from build123d import *

# Parameters (mm, degrees)
SKETCH_R          = 1.7
PAD_DEPTH         = 8
SKETCH001_R       = 1.5
POCKET_DEPTH      = 12.501
POCKET_DEPTH_BACK = -12.501
SKETCH002_R       = 3
POCKET001_DEPTH   = 2.25
SKETCH003_R       = 6
SKETCH003_R_2     = 3
POCKET002_DEPTH   = 4
SKETCH004_R       = 2.5
POCKET003_DEPTH   = 25.001
POCKET004_DEPTH   = 25.001
CHAMFER_SIZE      = 1
CHAMFER001_SIZE   = 1.5


with BuildPart() as part:
    # Sketch → Pad (new body)
    with BuildSketch(Plane.XY):
        Polygon((-12.5, 18), (-12.5, 0), (-12.5, -18), (0, -18), (12.5, -18), (12.5, 0), (12.5, 18), (0, 18), align=None)
        with Locations((6.5, -13)):
            Circle(SKETCH_R, mode=Mode.SUBTRACT)
        with Locations((-6.5, -13)):
            Circle(SKETCH_R, mode=Mode.SUBTRACT)
    extrude(amount=PAD_DEPTH)

    # Sketch001 → Pocket (cut, two sides)
    with BuildSketch(Plane.YZ) as pocket_sk:
        with Locations((0, 1.5)):
            Circle(SKETCH001_R)
    extrude(amount=-POCKET_DEPTH, mode=Mode.SUBTRACT)
    extrude(pocket_sk.sketch, amount=-POCKET_DEPTH_BACK, mode=Mode.SUBTRACT)

    # Sketch002 → Pocket001 (cut, symmetric)
    with BuildSketch(Plane.YZ):
        with Locations((0, 1.5)):
            Circle(SKETCH002_R)
    extrude(amount=POCKET001_DEPTH, both=True, mode=Mode.SUBTRACT)

    # Sketch003 → Pocket002 (cut, symmetric)
    with BuildSketch(Plane.YZ):
        with Locations((0, 1.5)):
            Circle(SKETCH003_R)
        with Locations((0, 1.5)):
            Circle(SKETCH003_R_2, mode=Mode.SUBTRACT)
    extrude(amount=POCKET002_DEPTH, both=True, mode=Mode.SUBTRACT)

    # Sketch004 (on DatumPlane) → Pocket003 (cut, through all)
    with BuildSketch(Plane(origin=(-12.5, 13, 8), x_dir=(0, -1, 0), z_dir=(-1, 0, 0))):
        Circle(SKETCH004_R)
    extrude(amount=-POCKET003_DEPTH, mode=Mode.SUBTRACT)

    # Sketch005 (on DatumPlane) → Pocket004 (cut, through all)
    with BuildSketch(Plane(origin=(-12.5, 13, 0), x_dir=(0, -1, 0), z_dir=(-1, 0, 0))):
        with BuildLine():
            ThreePointArc((-8, 8), (-5.656854, 2.343146), (0, 0))
            Line((0, 0), (0, -10))
            ThreePointArc((-18, 8), (-12.727922, -4.727922), (0, -10))
            Line((-8, 8), (-18, 8))
        make_face()
    extrude(amount=-POCKET004_DEPTH, mode=Mode.SUBTRACT)

    # Chamfer
    chamfer_edges = [part.edges().sort_by_distance(p)[0] for p in [
        (-4, -0.776457, 4.397777),
        (4, -0.776457, 4.397777),
    ]]
    chamfer(chamfer_edges, length=CHAMFER_SIZE)

    # Chamfer001
    chamfer001_edges = [part.edges().sort_by_distance(p)[0] for p in [
        (0, 5.809475, 0),
        (0, -5.809475, 0),
    ]]
    chamfer(chamfer001_edges, length=CHAMFER001_SIZE)


solid = part.part
The model under review builds one solid part; all positions refer to its coordinate system, in mm. A direction names the side the tool comes from. Round coordinates to 2 decimals unless told otherwise and drop trailing zeros. Loops run counter-clockwise (first coordinate to the right, second up) from the corner with the lowest first, then second, coordinate; pieces in that order, holes last. Notation, with made-up numbers: (-5, 10) -> (15, 10) arc R20 ccw to (15, 29) -> close; hole circle Ø9 at (39.5, 12.25). An arc over 180 degrees is marked (long way). Return JSON: item names as keys, results as strings.
(1) Add section D-D on y = 11. Write out the cut boundary in (x, z).
Solved:
{"outline": "(-12.5, 0) -> (12.5, 0) -> (12.5, 6.5) -> (-12.5, 6.5) -> close"}
(2) For faces 1 (the flat face through (2.25, 0, 3.3)), 2 (the conical face through (3.2, -0.1, 4.7)), 3 (the flat face through (0, -4, 8)), list the 3-axis set-ups (+Z, -Z, +X, -X, +Y, -Y) from which the entire face can be reached by the end or side of a thin tool; tool diameter is ignored.
Solved:
{"face 1": "-Z", "face 2": "none", "face 3": "+Z, +X, -X, +Y, -Y"}
(3) Add section C-C on y = -13. Write out the cut boundary in (x, z).
Solved:
{"outline": "(-12.5, 0) -> (-8.2, 0) -> (-8.2, 8) -> (-12.5, 8) -> close; (-4.8, 0) -> (4.8, 0) -> (4.8, 8) -> (-4.8, 8) -> close; (8.2, 0) -> (12.5, 0) -> (12.5, 8) -> (8.2, 8) -> close"}
(4) For line 1 (Y direction, x = -6.5, z = 4.75); line 2 (Y direction, x = 6.5, z = 6.25); line 3 (Y direction, x = 5.75, z = 1.75), list the stretches that pass through material, from the lowest coordinate up.
Solved:
{"line 1": "-18 to -14.7, -11.3 to 18", "line 2": "-18 to -14.7, -11.3 to 11.21, 14.79 to 18", "line 3": "-18 to -14.53, -11.47 to -1.48, 1.48 to 17.99"}
(5) For pin 1 (1.8 mm diameter, centred on y = 0, z = 1.5, fed in from +X), flat-tipped, find the tip position at first contact; note if it passes through.
Solved:
{"pin 1": "through"}
(6) The part is to be moulded in two halves that separate along Z. For faces 4 (the flat face through (0, -9, 0)), 5 (the flat face through (0, 17, 8)), 6 (the flat face through (4, -1, 6)), say which applies: released by +Z, released by -Z, zero draft, split by the parting line, or undercut.
Solved:
{"face 4": "released by -Z", "face 5": "released by +Z", "face 6": "undercut"}
